The model under review builds one solid part; all positions refer to its coordinate system, in mm. A direction names the side the tool comes from. Give positions to 0.01 mm unless a question says otherwise; leave off trailing zeros. Loops run counter-clockwise (first coordinate to the right, second up) from the corner with the lowest first, then second, coordinate; pieces in that order, holes last. Notation, with made-up numbers: M 39.25,30.25 L 81.25,30.25 A20 ccw 81.25,48.25 Z; hole C 60.5,26 d1. An arc over 180 degrees is marked long. Return JSON: item names as keys, results as strings.
```python
from build123d import *

# Parameters (mm, degrees)
SKETCH_1_W          = 38.4
SKETCH_1_H          = 4.8
SKETCH_1_R          = 0.95
EXTRUDE_1_DEPTH     = 4
EXTRUDE_2_DEPTH     = 21.2
SKETCH_5_R          = 7.8
CUT_EXTRUDE_2_DEPTH = 14.5
SKETCH_8_W          = 6
SKETCH_8_H          = 4.8
EXTRUDE_4_DEPTH     = 8
SKETCH_9_W          = 6
SKETCH_9_H          = 22
EXTRUDE_5_DEPTH     = 27.8


with BuildPart() as part:
    # 草图1 → 凸台-拉伸1 (new body)
    with BuildSketch(Plane.XY):
        with Locations((19.2, -2.4)):
            Rectangle(SKETCH_1_W, SKETCH_1_H)
        with Locations((10, -2.4)):
            Circle(SKETCH_1_R, mode=Mode.SUBTRACT)
        with Locations((28.4, -2.4)):
            Circle(SKETCH_1_R, mode=Mode.SUBTRACT)
    extrude(amount=EXTRUDE_1_DEPTH)

    # 草图4 → 凸台-拉伸2 (add)
    with BuildSketch(Plane(origin=(0, 0, 0), x_dir=(1, 0, 0), z_dir=(0, 1, 0))):
        Polygon((2.2, 0), (2.2, 4), (5.2, 4), (5.2, 10.5), (2.2, 10.5), (2.2, 14.5), (7.2, 14.5), (7.2, 0), align=None)
        Polygon((36.2, 0), (31.2, 0), (31.2, 14.5), (36.2, 14.5), (36.2, 10.5), (33.2, 10.5), (33.2, 4), (36.2, 4), align=None)
    extrude(amount=-EXTRUDE_2_DEPTH)

    # 草图5 → 切除-拉伸2 (cut)
    with BuildSketch(Plane(origin=(0, 0, -14.5), x_dir=(-1, 0, 0), z_dir=(0, 0, -1))):
        with Locations((-10, -21.2)):
            Circle(SKETCH_5_R)
        with Locations((-28.4, -21.2)):
            Circle(SKETCH_5_R)
    extrude(amount=-CUT_EXTRUDE_2_DEPTH, mode=Mode.SUBTRACT)

    # 草图8 → 凸台-拉伸4 (add)
    with BuildSketch(Plane.XY.offset(4)):
        with Locations((19.2, -2.4)):
            Rectangle(SKETCH_8_W, SKETCH_8_H)
    extrude(amount=EXTRUDE_4_DEPTH)

    # 草图9 → 凸台-拉伸5 (add)
    with BuildSketch(Plane.XZ.offset(4.8)):
        with Locations((19.2, 11)):
            Rectangle(SKETCH_9_W, SKETCH_9_H)
    extrude(amount=EXTRUDE_5_DEPTH)


solid = part.part
```
1) Consider section C-C on x = 10. Write out the cut boundary in (y, z).
From the geometry:
{"outline": "M -4.8,0 L -3.35,0 L -3.35,4 L -4.8,4 Z; M -1.45,0 L 0,0 L 0,4 L -1.45,4 Z"}
2) Wall thickness on L1, parallel to X at y = -2, z = -7.5; L2, parallel to X at y = -2, z = 2; L3, parallel to Z at x = 35, y = -9: over which ranges is each line inside the solid? List them lowest first. Write a range as from..to.
From the geometry:
{"L1": "5.2..7.2, 31.2..33.2", "L2": "0..9.14, 10.86..27.54, 29.26..38.4", "L3": "-14.5..-10.5, -4..0"}
3) The part is to be moulded in two halves that separate along Z. For faces 4 (the face through (35, -8, -10.5)), 5 (the face through (19, -12, 0)), 6 (the face through (35, -8, -4)), 7 (the face through (31.2, -7, -7)), say which applies: released by +Z, released by -Z, zero draft, split by the parting line, or undercut.
From the geometry:
{"face 4": "undercut", "face 5": "released by -Z", "face 6": "undercut", "face 7": "zero draft"}
4) Consider section A-A on y = -2.4. Count the separate pieces of the cut face and the enclosed holes in it, then the cut area to 3 significant figures.
From the geometry:
{"separate pieces": "3", "enclosed holes": "0", "area": "292 mm²"}
5) Consider section D-D on y = -17.5. Write out the cut boundary in (x, z), then the cut area to 3 significant figures.
From the geometry:
{"outline": "M 2.2,-14.5 L 3.13,-14.5 L 3.13,-10.5 L 2.2,-10.5 Z; M 2.2,-4 L 3.13,-4 L 3.13,0 L 2.2,0 Z; M 16.2,0 L 22.2,0 L 22.2,22 L 16.2,22 Z; M 35.27,-14.5 L 36.2,-14.5 L 36.2,-10.5 L 35.27,-10.5 Z; M 35.27,-4 L 36.2,-4 L 36.2,0 L 35.27,0 Z", "area": "147 mm²"}
6) Consider section B-B on z = -9. Write out the cut boundary in (x, y), then the cut area to 3 significant figures.
From the geometry:
{"outline": "M 5.2,-15.05 A7.8 cw 7.2,-13.92 L 7.2,0 L 5.2,0 Z; M 31.2,-13.92 A7.8 cw 33.2,-15.05 L 33.2,0 L 31.2,0 Z", "area": "57.7 mm²"}
7) Tool access review of faces 1 (the face through (36.2, -10, -2)), 2 (the face through (4, -8, -10.5)), 3 (the face through (2.2, -10, -2)): name each direction out of +Z, -Z, +X, -X, +Y, -Y from which nothing blocks a thin tool from reaching the whole face with its end or side.
From the geometry:
{"face 1": "-Z, +X, +Y, -Y", "face 2": "-X, +Y, -Y", "face 3": "-Z, -X, +Y, -Y"}
8) Insertion check: pin 1 (1 mm diameter, centred on x = 8, z = -3, fed in from +Y); pin 2 (7 mm diameter, centred on y = -10, z = -8.5, fed in from +X); pin 3 (2 mm diameter, centred on y = -14.5, z = -1, fed in from -X); pin 4 (1.4 mm diameter, centred on x = 20.5, y = -2, fed in from +Z). Each pin has a flat end and moves straight along its axis. Give the tip position at first contact, or say it passes through.
From the geometry:
{"pin 1": "through", "pin 2": "x = 36.2", "pin 3": "x = 2.2", "pin 4": "z = 12"}
